Design review of the part built by this model. Coordinates are the model's own, in mm. Round coordinates to 2 decimals unless told otherwise and drop trailing zeros. Order: outer loops, then holes, each group sorted by start corner. A loop starts at its lowest first (then second) coordinate and runs counter-clockwise, first axis right, second up. Notation, with made-up numbers: M -9,10.25 L 34,10.25 A25 cw 34,48.25 Z; hole C 49.5,38.5 d10. An arc over 180 degrees is marked long. Use a Markdown table: item, result. Add a question column.
(1) For pin 1 (9 mm diameter, centred on x = -10.56, y = -19.63, fed in from -Z); pin 2 (0.9 mm diameter, centred on y = -70, z = 1, fed in from -X); pin 3 (1.5 mm diameter, centred on y = -43, z = 1, fed in from +X), all flat-tipped, find the tip position at first contact; note any pin that passes through.
(2) To check wall thickness, follow probe 1 along Y at (x, z) = (0, 1.95); probe 2 along X at (y, z) = (-62, 0.25); probe 3 along Y at (x, z) = (10.56, 1.35). State the ranges of each line that lie inside material, in increasing order. Write a range as from..to.
(3) Take a section at D-D (z = 1.05). Count the separate pieces of the cut face and the enclosed holes in it, then the cut area to 3 significant figures.
(4) Take a section at A-A (x = 0). Write out the cut boundary in (y, z).
(5) Take a section at B-B (y = -71.5). Write out the cut boundary in (x, z), then the cut area to 3 significant figures.
(6) Take a section at C-C (x = -10.56). Write out the cut boundary in (y, z).
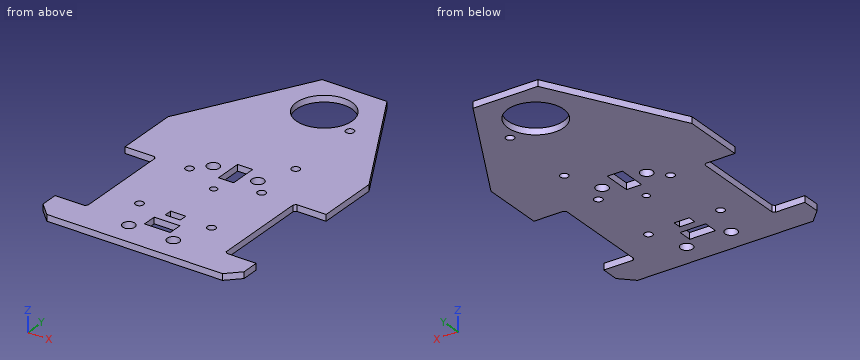
```python
from build123d import *

# Parameters (mm, degrees)
ESQUISSE1_R        = 13.2
ESQUISSE1_R_2      = 1.92
ESQUISSE1_R_3      = 2.88
ESQUISSE1_R_4      = 1.63358903
ESQUISSE1_W        = 7.152
ESQUISSE1_H        = 3.804
ESQUISSE1_W_2      = 7.15
ESQUISSE1_H_2      = 13.08
ESQUISSE1_W_3      = 12.18
ESQUISSE1_H_3      = 6.6
BOSS_EXTRU_1_DEPTH = 3


with BuildPart() as part:
    # Esquisse1 → Boss.-Extru.1 (new body)
    with BuildSketch(Plane.XY):
        Polygon((-15.36, 61.550503597), (15.36, 61.550503597), (47.64, 2.810503597), (47.64, -26.469496403), (33.76, -26.469496403), (32.76, -27.469496403), (32.76, -73.169496403), (33.76, -74.169496403), (47.64, -74.169496403), (47.64, -82.449496403), (41.64, -88.449496403), (-41.64, -88.449496403), (-47.64, -82.449496403), (-47.64, -74.169496403), (-33.76, -74.169496403), (-32.76, -73.169496403), (-32.76, -27.469496403), (-33.76, -26.469496403), (-47.64, -26.469496403), (-47.64, 2.810503597), align=None)
        with Locations((0, 40.850503597)):
            Circle(ESQUISSE1_R, mode=Mode.SUBTRACT)
        with Locations((17.076, -26.469496403)):
            Circle(ESQUISSE1_R_2, mode=Mode.SUBTRACT)
        with Locations((17.076, -60.621496403)):
            Circle(ESQUISSE1_R_2, mode=Mode.SUBTRACT)
        with Locations((10.56, -77.301496403)):
            Circle(ESQUISSE1_R_3, mode=Mode.SUBTRACT)
        with Locations((-10.56, -77.301496403)):
            Circle(ESQUISSE1_R_3, mode=Mode.SUBTRACT)
        with Locations((-17.076, -60.621496403)):
            Circle(ESQUISSE1_R_2, mode=Mode.SUBTRACT)
        with Locations((-17.076, -26.469496403)):
            Circle(ESQUISSE1_R_2, mode=Mode.SUBTRACT)
        with Locations((17.076, 33.802499019)):
            Circle(ESQUISSE1_R_2, mode=Mode.SUBTRACT)
        with Locations((17.076, -3.201200519)):
            Circle(ESQUISSE1_R_2, mode=Mode.SUBTRACT)
        with Locations((0, -34.547074796)):
            Circle(ESQUISSE1_R_4, mode=Mode.SUBTRACT)
        with Locations((10.56, -19.626900252)):
            Circle(ESQUISSE1_R_3, mode=Mode.SUBTRACT)
        with Locations((-10.56, -19.626900252)):
            Circle(ESQUISSE1_R_3, mode=Mode.SUBTRACT)
        with Locations((0, -60.627496403)):
            Rectangle(ESQUISSE1_W, ESQUISSE1_H, mode=Mode.SUBTRACT)
        with Locations((0, -19.629496403)):
            Rectangle(ESQUISSE1_W_2, ESQUISSE1_H_2, mode=Mode.SUBTRACT)
        with Locations((0, -69.669496403)):
            Rectangle(ESQUISSE1_W_3, ESQUISSE1_H_3, mode=Mode.SUBTRACT)
    extrude(amount=BOSS_EXTRU_1_DEPTH)


solid = part.part
```
Verdict:
| question | item | result |
|---|---|---|
| 1 | pin 1 | stops at z = 0 |
| 1 | pin 2 | stops at x = -32.76 |
| 1 | pin 3 | stops at x = 32.76 |
| 2 | probe 1 | y = -88.45..-72.97, -66.37..-62.53, -58.73..-36.18, -32.91..-26.17, -13.09..27.65, 54.05..61.55 |
| 2 | probe 2 | x = -32.76..-18.41, -15.74..-3.58, 3.58..15.74, 18.41..32.76 |
| 2 | probe 3 | y = -88.45..-80.18, -74.42..-22.51, -16.75..32.93, 48.77..61.55 |
| 3 | separate pieces | 1 |
| 3 | enclosed holes | 15 |
| 3 | area | 10,000 mm^2 |
| 4 | outline | M -88.45,0 L -72.97,0 L -72.97,3 L -88.45,3 Z; M -66.37,0 L -62.53,0 L -62.53,3 L -66.37,3 Z; M -58.73,0 L -36.18,0 L -36.18,3 L -58.73,3 Z; M -32.91,0 L -26.17,0 L -26.17,3 L -32.91,3 Z; M -13.09,0 L 27.65,0 L 27.65,3 L -13.09,3 Z; M 54.05,0 L 61.55,0 L 61.55,3 L 54.05,3 Z |
| 5 | outline | M -32.76,0 L -6.09,0 L -6.09,3 L -32.76,3 Z; M 6.09,0 L 32.76,0 L 32.76,3 L 6.09,3 Z |
| 5 | area | 160 mm^2 |
| 6 | outline | M -88.45,0 L -80.18,0 L -80.18,3 L -88.45,3 Z; M -74.42,0 L -22.51,0 L -22.51,3 L -74.42,3 Z; M -16.75,0 L 32.93,0 L 32.93,3 L -16.75,3 Z; M 48.77,0 L 61.55,0 L 61.55,3 L 48.77,3 Z |
